```python
from build123d import *

# Parameters (mm, degrees)
CYLINDER035_R          = 1.75
CYLINDER035_DEPTH      = 44
CYLINDER035_ROLL_ANGLE = 90
CYLINDER034_R          = 1.75
CYLINDER034_DEPTH      = 44
CYLINDER034_ROLL_ANGLE = 90
CYLINDER037_R          = 6
CYLINDER037_DEPTH      = 34
CYLINDER037_ROLL_ANGLE = 90
CYLINDER024_R          = 1.75
CYLINDER024_DEPTH      = 44
CYLINDER024_ROLL_ANGLE = 90
BOX054_W               = 37
BOX054_H               = 5
BOX054_DEPTH           = 14
BOX054_PITCH_ANGLE     = 18
BOX055_W               = 22
BOX055_H               = 5
BOX055_DEPTH           = 11
BOX055_PITCH_ANGLE     = -45
BOX056_W               = 12
BOX056_H               = 5
BOX056_DEPTH           = 31
CYLINDER025_R          = 1.75
CYLINDER025_DEPTH      = 44
CYLINDER025_ROLL_ANGLE = 90
BOX053_W               = 47
BOX053_H               = 5
BOX053_DEPTH           = 27
FILLET_R               = 3
BOX057_W               = 47
BOX057_H               = 5
BOX057_DEPTH           = 11


with BuildPart() as cylinder_for_hole_4_motherboard002:
    # Cylinder035 → Cylinder035 (new body)
    with BuildSketch(Plane.XY):
        Circle(CYLINDER035_R)
    extrude(amount=CYLINDER035_DEPTH)


with BuildPart() as cylinder_for_hole_4_motherboard002_1:
    # Cylinder035 roll: moved
    add(cylinder_for_hole_4_motherboard002.part.rotate(Axis((0, 0, 0), (1, 0, 0)), CYLINDER035_ROLL_ANGLE))


with BuildPart() as cylinder_for_hole_4_motherboard002_2:
    # Cylinder035 placement: moved
    add(cylinder_for_hole_4_motherboard002_1.part.moved(Location((20, 6, -13.5))))


with BuildPart() as cylinder_for_hole_3_motherboard002:
    # Cylinder034 → Cylinder034 (new body)
    with BuildSketch(Plane.XY):
        Circle(CYLINDER034_R)
    extrude(amount=CYLINDER034_DEPTH)


with BuildPart() as cylinder_for_hole_3_motherboard002_1:
    # Cylinder034 roll: moved
    add(cylinder_for_hole_3_motherboard002.part.rotate(Axis((0, 0, 0), (1, 0, 0)), CYLINDER034_ROLL_ANGLE))


with BuildPart() as cylinder_for_hole_3_motherboard002_2:
    # Cylinder034 placement: moved
    add(cylinder_for_hole_3_motherboard002_1.part.moved(Location((-20, 6, -13.5))))


with BuildPart() as jhead_hole:
    # Cylinder037 → Cylinder037 (new body)
    with BuildSketch(Plane.XY):
        Circle(CYLINDER037_R)
    extrude(amount=CYLINDER037_DEPTH)


with BuildPart() as jhead_hole_1:
    # Cylinder037 roll: moved
    add(jhead_hole.part.rotate(Axis((0, 0, 0), (1, 0, 0)), CYLINDER037_ROLL_ANGLE))


with BuildPart() as jhead_hole_2:
    # Cylinder037 placement: moved
    add(jhead_hole_1.part.moved(Location((4.5, 0, -4))))


with BuildPart() as jhead_lock_plate_holes:
    # Fusion016 base: copy of jhead hole
    add(jhead_hole_2.part)

    # Fusion016: union cylinder for hole 4 - Motherboard002, cylinder for hole 3 - Motherboard002
    add(cylinder_for_hole_4_motherboard002_2.part)
    add(cylinder_for_hole_3_motherboard002_2.part)


with BuildPart() as cylinder_for_hole_9_groovemount_l001:
    # Cylinder024 → Cylinder024 (new body)
    with BuildSketch(Plane.XY):
        Circle(CYLINDER024_R)
    extrude(amount=CYLINDER024_DEPTH)


with BuildPart() as cylinder_for_hole_9_groovemount_l001_1:
    # Cylinder024 roll: moved
    add(cylinder_for_hole_9_groovemount_l001.part.rotate(Axis((0, 0, 0), (1, 0, 0)), CYLINDER024_ROLL_ANGLE))


with BuildPart() as cylinder_for_hole_9_groovemount_l001_2:
    # Cylinder024 placement: moved
    add(cylinder_for_hole_9_groovemount_l001_1.part.moved(Location((-20, 6, -2.5))))


with BuildPart() as jhead_retention_plate_chamfer_l:
    # Box054 → Box054 (new body)
    with BuildSketch(Plane.XY):
        with Locations((18.5, 2.5)):
            Rectangle(BOX054_W, BOX054_H)
    extrude(amount=BOX054_DEPTH)


with BuildPart() as jhead_retention_plate_chamfer_l_1:
    # Box054 pitch: moved
    add(jhead_retention_plate_chamfer_l.part.rotate(Axis((0, 0, 0), (0, 1, 0)), BOX054_PITCH_ANGLE))


with BuildPart() as jhead_retention_plate_chamfer_l_2:
    # Box054 placement: moved
    add(jhead_retention_plate_chamfer_l_1.part.moved(Location((-32.5, -24, -17))))


with BuildPart() as jhead_retention_plate_chamfer_r:
    # Box055 → Box055 (new body)
    with BuildSketch(Plane.XY):
        with Locations((11, 2.5)):
            Rectangle(BOX055_W, BOX055_H)
    extrude(amount=BOX055_DEPTH)


with BuildPart() as jhead_retention_plate_chamfer_r_1:
    # Box055 pitch: moved
    add(jhead_retention_plate_chamfer_r.part.rotate(Axis((0, 0, 0), (0, 1, 0)), BOX055_PITCH_ANGLE))


with BuildPart() as jhead_retention_plate_chamfer_r_2:
    # Box055 placement: moved
    add(jhead_retention_plate_chamfer_r_1.part.moved(Location((16.5, -24, -27))))


with BuildPart() as jhead_retention_plate_slide_in_hole:
    # Box056 → Box056 (new body)
    with BuildSketch(Plane(origin=(-1.5, -24, -35), x_dir=(1, 0, 0), z_dir=(0, 0, 1))):
        with Locations((6, 2.5)):
            Rectangle(BOX056_W, BOX056_H)
    extrude(amount=BOX056_DEPTH)


with BuildPart() as jhead_retention_plate_holes:
    # Cylinder025 → Cylinder025 (new body)
    with BuildSketch(Plane.XY):
        Circle(CYLINDER025_R)
    extrude(amount=CYLINDER025_DEPTH)


with BuildPart() as jhead_retention_plate_holes_1:
    # Cylinder025 roll: moved
    add(jhead_retention_plate_holes.part.rotate(Axis((0, 0, 0), (1, 0, 0)), CYLINDER025_ROLL_ANGLE))


with BuildPart() as jhead_retention_plate_holes_2:
    # Cylinder025 placement: moved
    add(jhead_retention_plate_holes_1.part.moved(Location((20, 6, -2.5))))

    # Fusion015: union cylinder for hole 9 - Groovemount L001, jhead hole, jhead retention plate chamfer L, jhead retention plate chamfer R, jhead retention plate slide in hole
    add(cylinder_for_hole_9_groovemount_l001_2.part)
    add(jhead_hole_2.part)
    add(jhead_retention_plate_chamfer_l_2.part)
    add(jhead_retention_plate_chamfer_r_2.part)
    add(jhead_retention_plate_slide_in_hole.part)


with BuildPart() as fillet_body:
    # Box053 → Box053 (new body)
    with BuildSketch(Plane(origin=(-23.5, -24, -19), x_dir=(1, 0, 0), z_dir=(0, 0, 1))):
        with Locations((23.5, 2.5)):
            Rectangle(BOX053_W, BOX053_H)
    extrude(amount=BOX053_DEPTH)

    # Cut009: cut jhead retention plate holes
    add(jhead_retention_plate_holes_2.part, mode=Mode.SUBTRACT)

    # Fillet
    fillet_edges = [fillet_body.edges().sort_by_distance(p)[0] for p in [
        (-23.5, -21.5, 8),
        (-23.5, -21.5, -5.203806),
        (23.5, -21.5, 8),
        (-1.5, -21.5, -12.352039),
        (10.5, -21.5, -17.443651),
        (23.5, -21.5, -4.443651),
    ]]
    fillet(fillet_edges, radius=FILLET_R)


with BuildPart() as cut011:
    # Box057 → Box057 (new body)
    with BuildSketch(Plane(origin=(-23.5, -24, -18), x_dir=(1, 0, 0), z_dir=(0, 0, 1))):
        with Locations((23.5, 2.5)):
            Rectangle(BOX057_W, BOX057_H)
    extrude(amount=BOX057_DEPTH)

    # Cut010: cut Fillet body
    add(fillet_body.part, mode=Mode.SUBTRACT)


with BuildPart() as cut011_1:
    # Cut010 placement: moved
    add(cut011.part.moved(Location((0, 0, -1))))

    # Cut011: cut jhead lock plate holes
    add(jhead_lock_plate_holes.part, mode=Mode.SUBTRACT)


solid = cut011_1.part
```
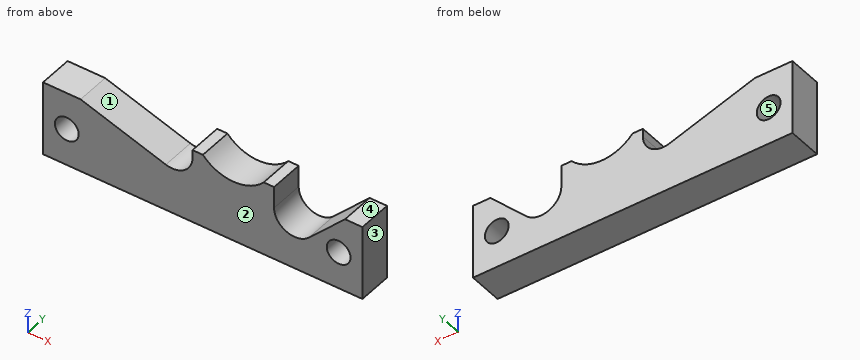
For this review, take the finished solid that the model builds, in its own axes (mm). Face numbers are marked on the shaded views. A direction names the side the tool comes from. Give positions to 0.01 mm unless a question says otherwise; leave off trailing zeros. Loops run counter-clockwise (first coordinate to the right, second up) from the corner with the lowest first, then second, coordinate; pieces in that order, holes last. Notation, with made-up numbers: M 15,-33.5 L 24,-33.5 A24 ccw 24,-1.5 Z; hole C 73,41.5 d3. An arc over 180 degrees is marked long. One line per item, written item: value. Start each with the question number.
Q1. Clearance check with flat-ended pins moving along their axes: pin 1 Ø1 at (x, z) = (15.5, -10) entering from +Y; pin 2 Ø4.5 at (x, z) = (20, -13.5) entering from -Y. State where each tip first meets the part, or that it passes through.
Q2. Add section B-B (y = -19.8). Give the boundary of the cut face in (x, z), and give its area (3 significant figures).
Q3. Add section C-C (z = -8.75). Give the boundary of the cut face in (x, y).
Q4. Draft analysis for pull direction Z (two halves, no side actions). For the marked faces 3, 4 and 5, state which applies: released by +Z, released by -Z, zero draft, split by the parting line, or undercut.
Q5. Machinability: for the marked faces 1 and 2, which of the approach directions +Z, -Z, +X, -X, +Y, -Y give a long, thin tool a straight path to every point of the face, cutting with its end or side? Answer none if there is none.
Q6. Add section A-A (x = -20). Give the boundary of the cut face in (y, z), and give its area (3 significant figures).
Q7. For L1, parallel to Z at x = -20, y = -21.5; L2, parallel to Z at x = 20, y = -22.9; L3, parallel to X at y = -23.75, z = -14.5, list the stretches that pass through material, from the lowest coordinate up.
Q8. Add section D-D (x = 20). Give the boundary of the cut face in (y, z).
Reply:
1. pin 1: through
1. pin 2: y = -24
2. outline: M -23.5,-19 L 23.5,-19 L 23.5,-8 L 20.94,-8 L 15.62,-13.32 A3 cw 10.5,-11.2 L 10.5,-8 L 8.97,-8 A6 cw 0.03,-8 L -1.5,-8 L -1.5,-9.22 A3 cw -5.43,-12.08 L -17.97,-8 L -23.5,-8 Z; hole C -20,-13.5 d3.5; hole C 20,-13.5 d3.5
2. area: 402 mm²
3. outline: M -23.5,-24 L -15.66,-24 L -15.66,-19 L -23.5,-19 Z; M -1.5,-24 L 0.83,-24 L 0.83,-19 L -1.5,-19 Z; M 8.17,-24 L 10.5,-24 L 10.5,-19 L 8.17,-19 Z; M 20.19,-24 L 23.5,-24 L 23.5,-19 L 20.19,-19 Z
4. face 3: zero draft
4. face 4: released by +Z
4. face 5: undercut
5. face 1: +Z, +Y, -Y
5. face 2: +Z, -Z, +X, -X, -Y
6. outline: M -24,-19 L -19,-19 L -19,-15.25 L -24,-15.25 Z; M -24,-11.75 L -19,-11.75 L -19,-8 L -24,-8 Z
6. area: 37.5 mm²
7. L1: -19 to -15.25, -11.75 to -8
7. L2: -19 to -15.25, -11.75 to -8.94
7. L3: -23.5 to -21.44, -18.56 to 18.56, 21.44 to 23.5
8. outline: M -24,-19 L -19,-19 L -19,-15.25 L -24,-15.25 Z; M -24,-11.75 L -19,-11.75 L -19,-8.94 L -24,-8.94 Z
